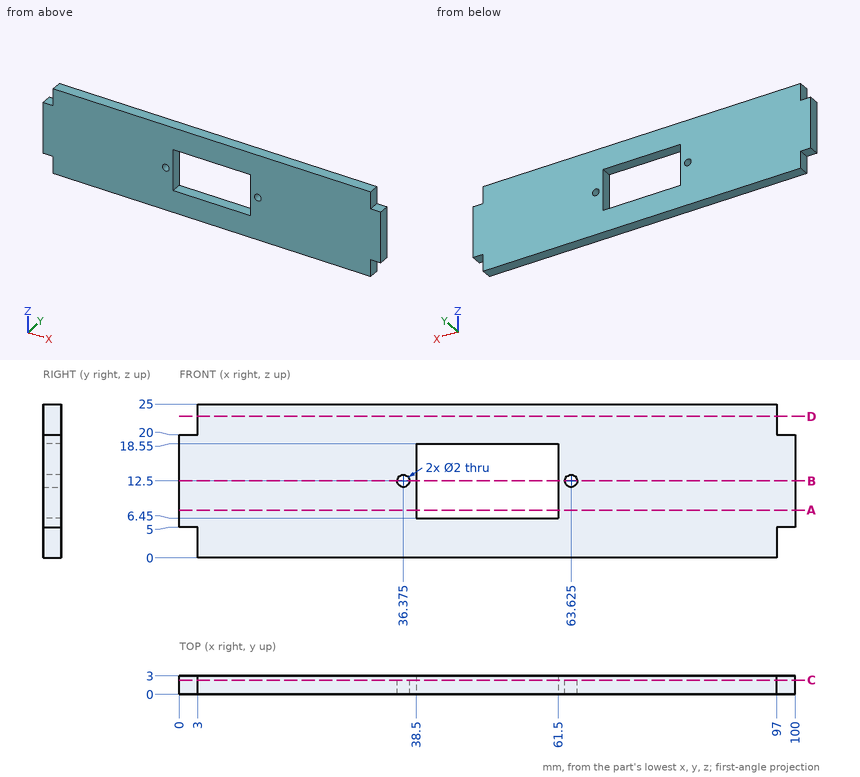
Can you work these out from the drawing? Everything is in mm from the part's minimum corner. Round coordinates to 2 decimals unless told otherwise and drop trailing zeros. Order: outer loops, then holes, each group sorted by start corner. A loop starts at its lowest first (then second) coordinate and runs counter-clockwise, first axis right, second up. Notation, with made-up numbers: (22.5, 18) -> (31.5, 18) arc R21 ccw to (31.5, 56) -> close; hole circle Ø4 at (25, 42). An arc over 180 degrees is marked (long way). Return JSON: item names as keys, results as strings. Group by question number.
1. If we section it at D-D, the plane z = 23: Write out the boundary of the cut face in (x, y), then the cut area to 3 significant figures.
2. If we section it at C-C, the plane y = 2.3: Write out the boundary of the cut face in (x, z) (3 decimals), then the cut area to 3 significant figures.
3. Will these pins go through, and if not, where does the flat tip stop? pin 1 (1.5 mm diameter, centred on x = 2, y = 1.5, fed in from +Z); pin 2 (1.5 mm diameter, centred on y = 2, z = 21.5, fed in from -X); pin 3 (1.5 mm diameter, centred on y = 1.5, z = 3.5, fed in from +X).
4. If we section it at B-B, the plane z = 12.5: Write out the boundary of the cut face in (x, y) (3 decimals).
5. If we section it at A-A, the plane z = 7.75: Write out the boundary of the cut face in (x, y), then the cut area to 3 significant figures.
6. I need wall thicknesses on line 1 (X direction, y = 1.4, z = 12.5) (3 decimals); line 2 (X direction, y = 0.25, z = 6.75); line 3 (Z direction, x = 45.5, y = 2.25). Which ranges of each line are inside material? Lowest first, please. Write a range as [from, to].
Output values:
{
 "1": {"outline": "(3, 0) -> (97, 0) -> (97, 3) -> (3, 3) -> close", "area": "282 mm²"},
 "2": {"outline": "(0, 5) -> (3, 5) -> (3, 0) -> (97, 0) -> (97, 5) -> (100, 5) -> (100, 20) -> (97, 20) -> (97, 25) -> (3, 25) -> (3, 20) -> (0, 20) -> close; hole circle Ø2 at (36.375, 12.5); hole (38.5, 6.45) -> (61.5, 6.45) -> (61.5, 18.55) -> (38.5, 18.55) -> close; hole circle Ø2 at (63.625, 12.5)", "area": "2,160 mm²"},
 "3": {"pin 1": "z = 20", "pin 2": "x = 3", "pin 3": "x = 97"},
 "4": {"outline": "(0, 0) -> (35.375, 0) -> (35.375, 3) -> (0, 3) -> close; (37.375, 0) -> (38.5, 0) -> (38.5, 3) -> (37.375, 3) -> close; (61.5, 0) -> (62.625, 0) -> (62.625, 3) -> (61.5, 3) -> close; (64.625, 0) -> (100, 0) -> (100, 3) -> (64.625, 3) -> close"},
 "5": {"outline": "(0, 0) -> (38.5, 0) -> (38.5, 3) -> (0, 3) -> close; (61.5, 0) -> (100, 0) -> (100, 3) -> (61.5, 3) -> close", "area": "231 mm²"},
 "6": {"line 1": "[0, 35.375], [37.375, 38.5], [61.5, 62.625], [64.625, 100]", "line 2": "[0, 38.5], [61.5, 100]", "line 3": "[0, 6.45], [18.55, 25]"}
}
